```python
from build123d import *

# Parameters (mm, degrees)
SKETCH_1_R      = 4
EXTRUDE_1_DEPTH = 3
SKETCH_2_W      = 3.2
SKETCH_2_H      = 3.2
EXTRUDE_3_DEPTH = 5


with BuildPart() as part:
    # Эскиз1 → Бобышка-Вытянуть1 (new body)
    with BuildSketch(Plane(origin=(0, 0, 0), x_dir=(1, 0, 0), z_dir=(0, 1, 0))):
        with Locations(Location((0, 0, 0), (0, 0, 270))):
            Circle(SKETCH_1_R)
    extrude(amount=EXTRUDE_1_DEPTH)

    # Эскиз2 → Бобышка-Вытянуть3 (add)
    with BuildSketch(Plane(origin=(0, 3, 0), x_dir=(1, 0, 0), z_dir=(0, 1, 0))):
        Rectangle(SKETCH_2_W, SKETCH_2_H)
    extrude(amount=EXTRUDE_3_DEPTH)


solid = part.part
```
Can you work these out from the model? Positions are in its coordinate system, mm. A direction names the side the tool comes from. Round coordinates to 2 decimals unless told otherwise and drop trailing zeros. Order: outer loops, then holes, each group sorted by start corner. A loop starts at its lowest first (then second) coordinate and runs counter-clockwise, first axis right, second up. Notation, with made-up numbers: (-23.5, -0.75) -> (-7.5, -0.75) arc R11 cw to (-7.5, 8.25) -> close; hole circle Ø10 at (20.5, 14.25). An arc over 180 degrees is marked (long way). Return JSON: item names as keys, results as strings. Group by question number.
1. If we section it at A-A, the plane z = 0: Write out the boundary of the cut face in (x, y).
2. If we section it at C-C, the plane y = 1.5: Write out the boundary of the cut face in (x, z).
3. If we section it at D-D, the plane y = 6: Write out the boundary of the cut face in (x, z), then the cut area to 3 significant figures.
4. Will these pins go through, and if not, where does the flat tip stop? pin 1 (1 mm diameter, centred on x = 0, y = 6.5, fed in from +Z); pin 2 (3 mm diameter, centred on y = 3, z = 2, fed in from +X); pin 3 (1 mm diameter, centred on y = 5.5, z = 0, fed in from +X).
5. Which directions (+Z, -Z, +X, -X, +Y, -Y) give clear straight access to the entire face, cutting with the end or side of a thin tool? Please do faces 1 (the face through (0, 0, 0)), 2 (the face through (0, 5, 1.6)), 3 (the face through (0, 5, -1.6)), 4 (the face through (1.6, 5, 0)), 5 (the face through (-1.6, 5, 0)).
6. If we section it at B-B, the plane x = 0: Write out the boundary of the cut face in (y, z).
7. I need wall thicknesses on line 1 (Z direction, x = 0, y = 4); line 2 (Y direction, x = -0.25, z = -2.75). Which ranges of each line are inside material? Lowest first, please. Write a range as [from, to].
Output values:
{
 "1": {"outline": "(-4, 0) -> (4, 0) -> (4, 3) -> (1.6, 3) -> (1.6, 8) -> (-1.6, 8) -> (-1.6, 3) -> (-4, 3) -> close"},
 "2": {"outline": "circle Ø8 at (0, 0)"},
 "3": {"outline": "(-1.6, -1.6) -> (1.6, -1.6) -> (1.6, 1.6) -> (-1.6, 1.6) -> close", "area": "10.2 mm²"},
 "4": {"pin 1": "z = 1.6", "pin 2": "x = 3.97", "pin 3": "x = 1.6"},
 "5": {"face 1": "+Z, -Z, +X, -X, -Y", "face 2": "+Z, +X, -X, +Y", "face 3": "-Z, +X, -X, +Y", "face 4": "+Z, -Z, +X, +Y", "face 5": "+Z, -Z, -X, +Y"},
 "6": {"outline": "(0, -4) -> (3, -4) -> (3, -1.6) -> (8, -1.6) -> (8, 1.6) -> (3, 1.6) -> (3, 4) -> (0, 4) -> close"},
 "7": {"line 1": "[-1.6, 1.6]", "line 2": "[0, 3]"}
}
